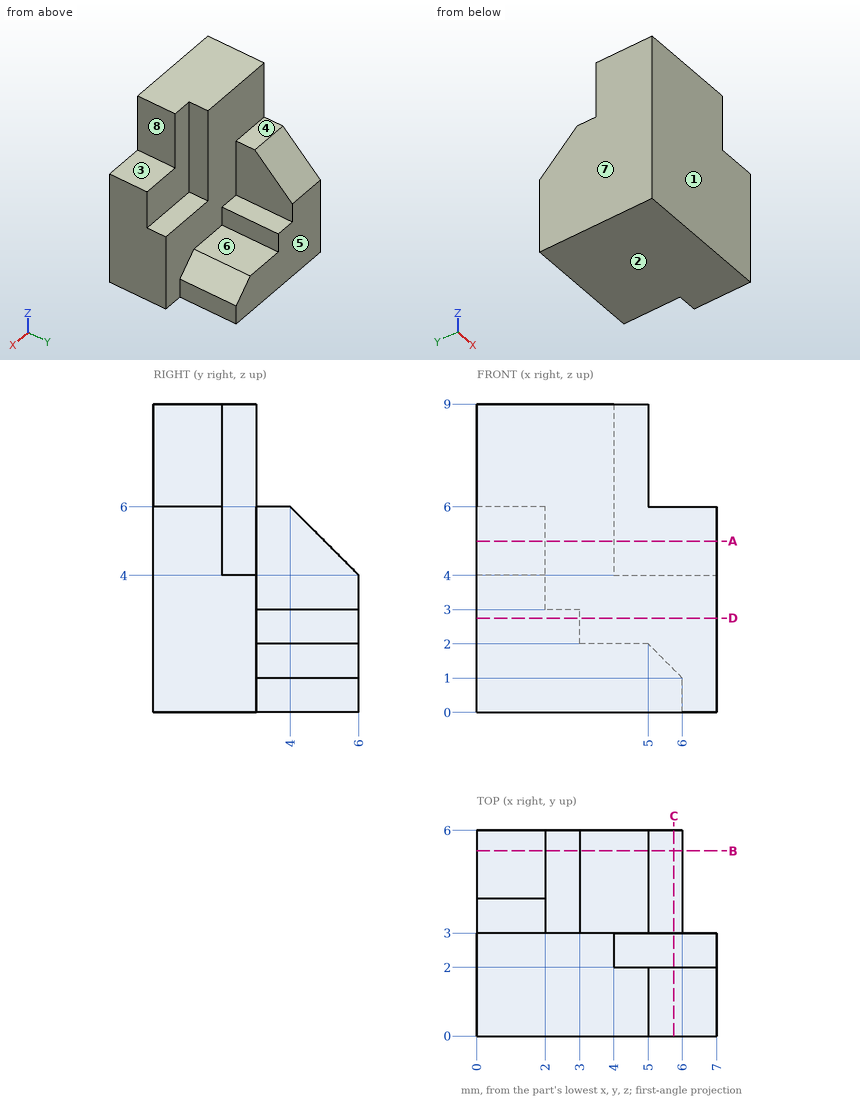
Answer from the drawing. Dimensions are ordinates in mm from the lowest x, y and z of the part. A direction names the side the tool comes from. Coordinates: 2 decimals unless noted, no trailing zeros. Write each loop counter-clockwise with the first axis right and the second up, starting at its lowest first coordinate (ties: lowest second). Pieces come first, ordered by that corner, then holes. Notation, with made-up numbers: (16, 54) - (41, 54) arc R33 ccw to (41, 87) - close; hole circle Ø7 at (88.5, 39.5). An arc over 180 degrees is marked (long way). Answer as CSV lines item,"result".
1. Straight lines are drawn through the part: line 1 (X direction, y = 2.55, z = 5.5); line 2 (X direction, y = 5.25, z = 2.5). For each, find the intervals that lie inside material, in ascending order. Write a range as [from, to].
Computed values:
line 1,"x = [0, 4]"
line 2,"x = [0, 3]"
2. Given P1, Ø0.5, axis at x = 6, y = 2.5, coming from the +Z side; P2, Ø1, axis at x = 6.5, y = 1, coming from the +Z side; P3, Ø0.8, axis at y = 2.5, z = 7.5, coming from the +X side, each flat-ended and moving along its own axis, determine where each tip first touches the part or whether it passes through.
Computed values:
P1,"stops at z = 4"
P2,"stops at z = 6"
P3,"stops at x = 4"
3. A tool of negligible diameter and unlimited length cuts with its end or side. For the marked faces 4, 5, 6, 7 and 8, from which of +Z, -Z, +X, -X, +Y, -Y can it reach the whole face along a straight path? Write none if from no direction.
Computed values:
face 4,"+Z, +X, -X, +Y"
face 5,"+Z, -Z, +X, -X, +Y"
face 6,"+Z, +X, +Y"
face 7,"+Z, -Z, -X, +Y, -Y"
face 8,"+Z, +X, +Y, -Y"
4. Find section C-C (x = 5.75). Give the vertices of the cut face in (y, z), plus the area to 4 significant figures.
Computed values:
outline,"(0, 0) - (6, 0) - (6, 1.25) - (3, 1.25) - (3, 4) - (2, 4) - (2, 6) - (0, 6) - close"
area,"19.75 mm²"
5. Find section D-D (z = 2.75). Give the vertices of the cut face in (x, y).
Computed values:
outline,"(0, 0) - (7, 0) - (7, 3) - (3, 3) - (3, 6) - (0, 6) - close"
6. Find section A-A (z = 5). Give the vertices of the cut face in (x, y), plus the area to 3 significant figures.
Computed values:
outline,"(0, 0) - (7, 0) - (7, 2) - (4, 2) - (4, 3) - (2, 3) - (2, 5) - (0, 5) - close"
area,"22.0 mm²"
7. Find section B-B (y = 5.4). Give the vertices of the cut face in (x, z), plus the area to 3 significant figures.
Computed values:
outline,"(0, 0) - (6, 0) - (6, 1) - (5, 2) - (3, 2) - (3, 3) - (2, 3) - (2, 4.6) - (0, 4.6) - close"
area,"17.7 mm²"
8. Determine the mould class of the marked faces 1, 2 and 3 for opening direction Z: +Z half, -Z half, draft (parallel to the pull), parting line (faces both ways), or undercut.
Computed values:
face 1,"draft"
face 2,"-Z half"
face 3,"+Z half"
